from build123d import *

# Parameters (mm, degrees)
F0_W     = 73.406
F0_H     = 28.575
F2_DEPTH = 7.112
F3_DEPTH = 6.35
F1_W     = 6.35
F1_H     = 28.575
F4_DEPTH = 6.3754
F5_DEPTH = 7.874


with BuildPart() as f2:
    # F0 (on Top) → F2 (new body, symmetric)
    with BuildSketch(Plane.XY):
        Rectangle(F0_W, F0_H)
    extrude(amount=F2_DEPTH, both=True)

    # F1 (on Top) → F3 (join, symmetric)
    with BuildSketch(Plane.XY):
        Polygon((-30.353, 42.8625), (-30.353, 14.2875), (36.703, 14.2875), (48.78324, 25.3365), (32.893, 25.3365), (32.893, 42.8625), align=None)
        with BuildLine():
            ThreePointArc((-20.270586, 24.638), (-25.858586, 30.226), (-20.270586, 35.814))
            Line((-20.270586, 35.814), (3.605414, 35.814))
            ThreePointArc((3.605414, 35.814), (9.193414, 30.226), (3.605414, 24.638))
            Line((3.605414, 24.638), (-20.270586, 24.638))
        make_face(mode=Mode.SUBTRACT)
        Polygon((36.703, -14.2875), (-30.353, -14.2875), (-30.353, -42.8625), (32.893, -42.8625), (32.893, -25.3365), (48.78324, -25.3365), align=None)
        with BuildLine():
            ThreePointArc((-20.270586, -35.814), (-25.858586, -30.226), (-20.270586, -24.638))
            Line((-20.270586, -24.638), (3.605414, -24.638))
            ThreePointArc((3.605414, -24.638), (9.193414, -30.226), (3.605414, -35.814))
            Line((3.605414, -35.814), (-20.270586, -35.814))
        make_face(mode=Mode.SUBTRACT)
    extrude(amount=F3_DEPTH, both=True)

    # F1 (on Top) → F4 (join)
    with BuildSketch(Plane.XY):
        with Locations((-33.528, -28.575)):
            Rectangle(F1_W, F1_H)
        with Locations((-33.528, 28.575)):
            Rectangle(F1_W, F1_H)
    extrude(amount=-F4_DEPTH)

    # F1 (on Top) → F5 (join, symmetric)
    with BuildSketch(Plane.XY):
        Polygon((32.893, -25.3365), (32.893, -42.8625), (67.945, -42.8625), (48.78324, -25.3365), align=None)
        Polygon((67.945, 42.8625), (32.893, 42.8625), (32.893, 25.3365), (48.78324, 25.3365), align=None)
    extrude(amount=F5_DEPTH, both=True)


solid = f2.part
The listing builds one solid part. Answer for the finished solid, in the listing's coordinates (mm). A direction names the side the tool comes from. Coordinates: 2 decimals unless noted, no trailing zeros. Loops run counter-clockwise (first coordinate to the right, second up) from the corner with the lowest first, then second, coordinate; pieces in that order, holes last. Notation, with made-up numbers: M 40,-20 L 74,-20 A30 cw 74,19 Z; hole C -34.5,63.5 d3. An arc over 180 degrees is marked long. Answer in a Markdown table with one row per item.
1) Given pin 1 (1.7 mm diameter, centred on y = -30, z = 7.5, fed in from -X); pin 2 (4 mm diameter, centred on x = 9.5, y = -4, fed in from +Z); pin 3 (8 mm diameter, centred on y = -19, z = 5, fed in from -X), each flat-ended and moving along its own axis, determine where each tip first touches the part or whether it passes through.
Answers below:
| item | result |
|---|---|
| pin 1 | x = 32.89 |
| pin 2 | z = 7.11 |
| pin 3 | x = -30.35 |
2) Which of the six approach directions +Z, -Z, +X, -X, +Y, -Y give full straight-line access (tool end or side, diameter ignored) to faces 3 (the flat face through (-34, -28, -6.375)), 4 (the flat face through (-34, 29, -6.375)), 5 (the cylindrical face through (9.19, -30.1, 0.09))?
Answers below:
| item | result |
|---|---|
| face 3 | -Z, -X, -Y |
| face 4 | -Z, -X, +Y |
| face 5 | +Z, -Z |
3) Find the intervals of material crossed by probe 1 along Y at (x, z) = (-14, -1); probe 2 along Y at (x, z) = (41.5, -6.75); probe 3 along Y at (x, z) = (22.5, -6.5), in increasing order.
Answers below:
| item | result |
|---|---|
| probe 1 | -42.86 to -35.81, -24.64 to 24.64, 35.81 to 42.86 |
| probe 2 | -42.86 to -25.34, 25.34 to 42.86 |
| probe 3 | -14.29 to 14.29 |
4) Determine the mould class of faces 1 (the flat face through (-8, -24.638, 0)), 2 (the flat face through (-30.353, -28, 3)) for opening direction X: released by +X, released by -X, zero draft, split by the parting line, or undercut.
Answers below:
| item | result |
|---|---|
| face 1 | undercut |
| face 2 | released by -X |
5) Find section A-A (x = -2). Determine the outline of the cut face in (y, z).
Answers below:
| item | result |
|---|---|
| outline | M -42.86,-6.35 L -35.81,-6.35 L -35.81,6.35 L -42.86,6.35 Z; M -24.64,-6.35 L -14.29,-6.35 L -14.29,-7.11 L 14.29,-7.11 L 14.29,-6.35 L 24.64,-6.35 L 24.64,6.35 L 14.29,6.35 L 14.29,7.11 L -14.29,7.11 L -14.29,6.35 L -24.64,6.35 Z; M 35.81,-6.35 L 42.86,-6.35 L 42.86,6.35 L 35.81,6.35 Z |
6) Find section C-C (x = 30.5). Determine the outline of the cut face in (y, z).
Answers below:
| item | result |
|---|---|
| outline | M -42.86,-6.35 L -14.29,-6.35 L -14.29,-7.11 L 14.29,-7.11 L 14.29,-6.35 L 42.86,-6.35 L 42.86,6.35 L 14.29,6.35 L 14.29,7.11 L -14.29,7.11 L -14.29,6.35 L -42.86,6.35 Z |
7) Find section B-B (z = -1.75). Determine the outline of the cut face in (x, y) (1 decimal), then the cut area to 3 significant figures.
Answers below:
| item | result |
|---|---|
| outline | M -36.7,-42.9 L 67.9,-42.9 L 36.7,-14.3 L 36.7,14.3 L 67.9,42.9 L -36.7,42.9 Z; hole M -20.3,-35.8 L 3.6,-35.8 A5.6 ccw 3.6,-24.6 L -20.3,-24.6 A5.6 ccw Z; hole M -20.3,24.6 L 3.6,24.6 A5.6 ccw 3.6,35.8 L -20.3,35.8 A5.6 ccw Z |
| area | 6,460 mm^2 |
